Could you check a few things on this model? Use its own coordinates, in mm. Face numbers are marked on the shaded views. Give positions to 0.01 mm unless a question says otherwise; leave off trailing zeros. Write each loop counter-clockwise with the first axis right and the second up, starting at its lowest first coordinate (ties: lowest second). Pieces come first, ordered by that corner, then holes. Notation, with made-up numbers: (-12, 69.25) - (35, 69.25) arc R26 ccw to (35, 102.25) - close; hole circle Ø8 at (19, 15). An arc over 180 degrees is marked (long way). Write item = value, one per line.
from build123d import *

# Parameters (mm, degrees)
F0_R     = 8.25
F0_R_2   = 4
F1_DEPTH = 2
F2_DEPTH = 2


# Not quite as in the source:
# - a fillet or chamfer that OpenCascade refuses, or shapes differently, is made with other operations: its cross-section is extruded or revolved along the edge and cut away or added


with BuildPart() as f1:
    # F0 (on Top) → F1 (new body)
    with BuildSketch(Plane.XY):
        Circle(F0_R)
        Circle(F0_R_2, mode=Mode.SUBTRACT)
        Circle(F0_R_2)
    extrude(amount=F1_DEPTH)

    # F0 (on Top) → F2 (cut, through all)
    with BuildSketch(Plane.XY):
        Circle(F0_R_2)
    extrude(amount=F2_DEPTH, mode=Mode.SUBTRACT)

    # F3: fillet of radius 3 on 1 edges, made by hand

    # F3_s1 → F3_t2 (revolve, cut)
    with BuildSketch(Plane.XZ):
        with BuildLine():
            ThreePointArc((8.25, 0), (7.1536236828, 1.4494897428), (5.4215728753, 2))
            Line((5.4215728753, 2), (8.25, 2))
            Line((8.25, 2), (8.25, 0))
        make_face()
    revolve(axis=Axis((0, 0, 2), (0, 0, 1)), mode=Mode.SUBTRACT)


solid = f1.part
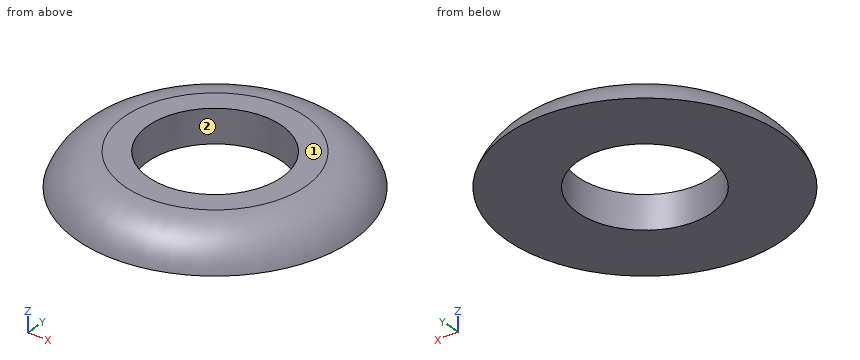
1. I need wall thicknesses on line 1 (Y direction, x = 0, z = 1.1); line 2 (X direction, y = 2, z = 1.1); line 3 (Y direction, x = 0, z = 1.45). Which ranges of each line are inside material? Lowest first, please.
Filled sheet:
line_1 = -7.56 to -4, 4 to 7.56
line_2 = -7.29 to -3.46, 3.46 to 7.29
line_3 = -7.15 to -4, 4 to 7.15
2. Thinking about a two-plate mould opening in Y: for the marked faces 1 and 2, which applies, pulls with the +Y half, pulls with the -Y half, needs draft (parallel to the pull), parting line crosses it, or undercut?
Filled sheet:
face_1 = needs draft
face_2 = undercut
3. For pin 1 (3 mm diameter, centred on x = -2.5, y = -6, fed in from -Z); pin 2 (1 mm diameter, centred on y = 1.5, z = 1.5, fed in from +X), each with a flat end and sliding along its axis, tell me the tip position at first contact or that it passes through.
Filled sheet:
pin_1 = 0
pin_2 = 7.52
4. If we section it at D-D, the plane z = 1.5: Please give me the cut outline in (x, y), and give its area (3 significant figures).
Filled sheet:
outline = circle Ø14.16 at (0, 0); hole circle Ø8 at (0, 0)
area = 107 mm2
5. If we section it at C-C, the plane z = 0.6: Please give me the cut outline in (x, y), and give its area (3 significant figures).
Filled sheet:
outline = circle Ø15.92 at (0, 0); hole circle Ø8 at (0, 0)
area = 149 mm2
6. If we section it at A-A, the plane x = 0: Please give me the cut outline in (y, z), and give its area (3 significant figures).
Filled sheet:
outline = (-8.25, 0) - (-4, 0) - (-4, 2) - (-5.42, 2) arc R3 ccw to start; (4, 0) - (8.25, 0) arc R3 ccw to (5.42, 2) - (4, 2) - close
area = 13.9 mm2
